Design review of the part built by this model. Coordinates are the model's own, in mm. Face numbers are marked on the shaded views. Coordinates: 2 decimals unless noted, no trailing zeros. Loops run counter-clockwise (first coordinate to the right, second up) from the corner with the lowest first, then second, coordinate; pieces in that order, holes last. Notation, with made-up numbers: (24.25, 33) -> (62.25, 33) arc R35 cw to (62.25, 67) -> close; hole circle Ø7 at (77, 30). An arc over 180 degrees is marked (long way). One line per item, written item: value. Start each with the question number.
1. Insertion check: pin 1 (10 mm diameter, centred on x = 793, y = 733, fed in from +Z) (3 decimals); pin 2 (1 mm diameter, centred on x = 802.5, z = 5.5, fed in from -Y); pin 3 (5 mm diameter, centred on y = 730, z = 2, fed in from -X); pin 4 (4 mm diameter, centred on y = 720, z = 5.5, fed in from -X). Each pin has a flat end and moves straight along its axis. Give the tip position at first contact, or say it passes through.
2. Add section A-A on y = 722. Give the number of separate pieces and of enclosed holes in the cut face, plus the area to 3 significant figures.
3. Add section B-B on x = 820. Write out the cut boundary in (y, z) (1 decimal), plus the area to 3 significant figures.
4. Draft analysis for pull direction X (two halves, no side actions). For the marked faces 1, 2, 3 and 4, state which applies: pulls with the +X half, pulls with the -X half, needs draft (parallel to the pull), parting line crosses it, or undercut.
5. For probe 1 along X at (y, z) = (734, 5.25); probe 2 along Y at (x, z) = (808.5, 6.25); probe 3 along Y at (x, z) = (807.5, 9.25), list the stretches that pass through material, from the lowest coordinate up.
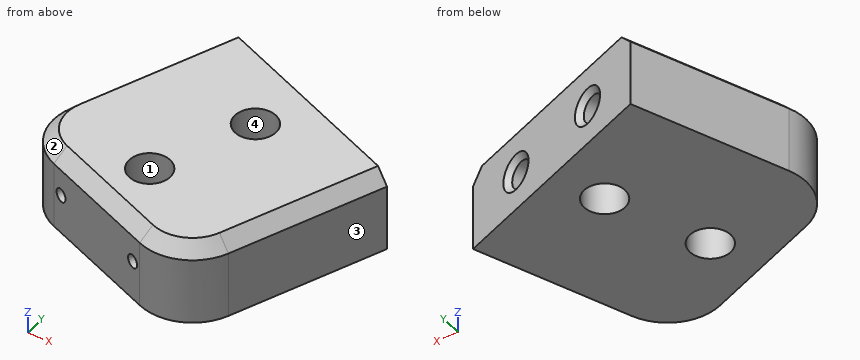
```python
from build123d import *

# Parameters (mm, degrees)
BOSS_EXTRUDE1_DEPTH                 = 9.525
FILLET1_R                           = 6.35
CHAMFER3_SIZE                       = 1.5875
F_1_8_0_126_DOWEL_HOLE1_D           = 3.2004
F_1_8_0_126_DOWEL_HOLE1_DEPTH       = 11.1125
F_1_8_0_126_DOWEL_HOLE1_CSINK_D     = 4.4704
F_1_8_0_126_DOWEL_HOLE1_CSINK_ANGLE = 90
F_1_8_0_126_DOWEL_HOLE1_TIP         = 0.961497163
F_1_16_0_0625_DIAMETER_HOLE1_D      = 1.5875
F_8_CLEARANCE_HOLE1_D               = 4.9149


with BuildPart() as part:
    # Sketch1 → Boss-Extrude1 (new body)
    with BuildSketch(Plane.XY):
        Polygon((822.963473633, 732.863646666), (813.457215496, 709.309643689), (787.547812221, 719.76652764), (797.054070358, 743.320530617), align=None)
    extrude(amount=BOSS_EXTRUDE1_DEPTH)

    # Fillet1
    fillet1_edges = [part.edges().sort_by_distance(p)[0] for p in [
        (813.457215496, 709.309643689, 4.7625),
        (787.547812221, 719.76652764, 4.7625),
    ]]
    fillet(fillet1_edges, radius=FILLET1_R)

    # Chamfer3
    chamfer3_edges = [part.edges().sort_by_distance(p)[0] for p in [
        (800.502513859, 714.538085664, 9.525),
        (819.398626831, 724.03089555, 9.525),
        (812.428593195, 711.730425262, 9.525),
        (789.968593794, 720.795149941, 9.525),
        (793.489223557, 734.4877795, 9.525),
    ]]
    chamfer(chamfer3_edges, length=CHAMFER3_SIZE)

    # 1/8 (0.126) Dowel Hole1
    with Locations(Plane(origin=(369.623280938, 915.829102682, 0), x_dir=(0.9273229518431505, -0.3742621313797403, 0), z_dir=(0.3742621313797403, 0.9273229518431505, 0))):
        with Locations((481.249807216, -4.7625), (468.549807216, -4.7625)):
            CounterSinkHole(F_1_8_0_126_DOWEL_HOLE1_D / 2, F_1_8_0_126_DOWEL_HOLE1_CSINK_D / 2, depth=F_1_8_0_126_DOWEL_HOLE1_DEPTH, counter_sink_angle=F_1_8_0_126_DOWEL_HOLE1_CSINK_ANGLE)
            with Locations((0, 0, -(F_1_8_0_126_DOWEL_HOLE1_DEPTH + F_1_8_0_126_DOWEL_HOLE1_TIP / 2))):  # 118° drill point
                Cone(0, F_1_8_0_126_DOWEL_HOLE1_D / 2, F_1_8_0_126_DOWEL_HOLE1_TIP, mode=Mode.SUBTRACT)

    # 1/16 (0.0625) Diameter Hole1 (through all)
    with Locations(Plane(origin=(369.623280938, 915.829102682, 0), x_dir=(0.9273229518431505, -0.3742621313797403, 0), z_dir=(0.3742621313797403, 0.9273229518431505, 0))):
        with Locations((468.549807216, -4.7625), (481.249807216, -4.7625)):
            Hole(F_1_16_0_0625_DIAMETER_HOLE1_D / 2)

    # #8 Clearance Hole1 (through all)
    with Locations(Plane.XY.offset(9.525)):
        with Locations((802.879078393, 720.426586409), (807.632207461, 732.203587897)):
            Hole(F_8_CLEARANCE_HOLE1_D / 2)


solid = part.part
```
Worked answers:
1. pin 1: stops at z = 9.525
1. pin 2: stops at y = 713.53
1. pin 3: stops at x = 790.67
1. pin 4: stops at x = 789.59
2. separate pieces: 2
2. enclosed holes: 2
2. area: 233 mm²
3. outline: (725.5, 0) -> (734.1, 0) -> (734.1, 9.5) -> (729.8, 9.5) -> (725.5, 7.9) -> close
3. area: 78.0 mm²
4. face 1: undercut
4. face 2: pulls with the -X half
4. face 3: pulls with the +X half
4. face 4: undercut
5. probe 1: x = 793.29 to 799.87, 803.15 to 805.96, 809.31 to 813.56, 816.85 to 820.15
5. probe 2: y = 711.39 to 729.9, 734.5 to 738.7
5. probe 3: y = 713.13 to 729.75, 734.66 to 739.1
